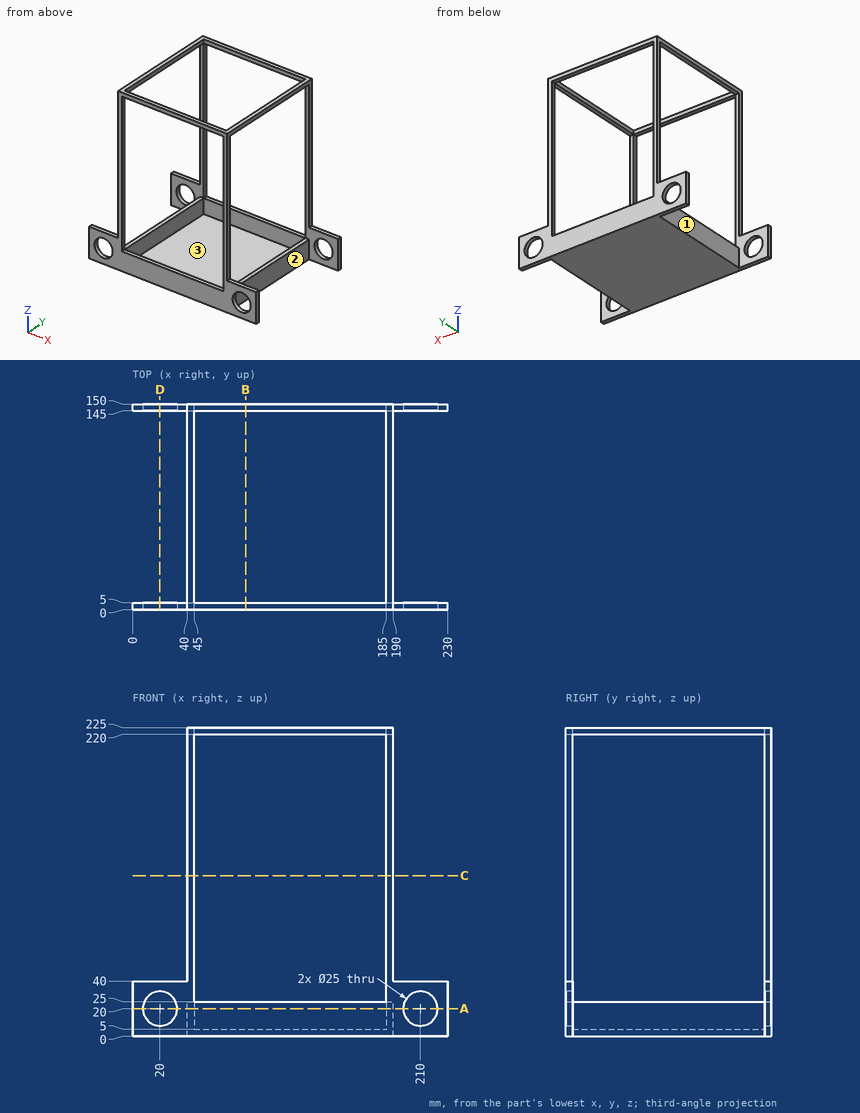
The drawing under review shows one solid part. Ordinate dimensions are in mm from its lowest x, y, z. Coordinates: 2 decimals unless noted, no trailing zeros. Loops run counter-clockwise (first coordinate to the right, second up) from the corner with the lowest first, then second, coordinate; pieces in that order, holes last. Notation, with made-up numbers: M 84.25,27.25 L 109.25,27.25 A22 ccw 109.25,56.25 Z; hole C -15.5,86 d11. An arc over 180 degrees is marked long. Use one line per item in the form item = value.
(1) For line 1 along X through (y, z) = (1, 20); line 2 along X through (y, z) = (55, 18.5); line 3 along Y through (x, z) = (73.5, 15.5), list the stretches that pass through material, from the lowest coordinate up. Write a range as from..to.
Return value:
line_1 = 0..7.5, 32.5..197.5, 222.5..230
line_2 = 40..45, 185..190
line_3 = 0..5, 145..150
(2) Consider section A-A (z = 20). Give the number of separate pieces and of enclosed holes in the cut face, and give its area (3 significant figures).
Return value:
separate_pieces = 5
enclosed_holes = 1
area = 3,200 mm2
(3) Consider section C-C (z = 117). Write out the cut boundary in (x, y), and give its area (3 significant figures).
Return value:
outline = M 40,0 L 45,0 L 45,5 L 40,5 Z; M 40,145 L 45,145 L 45,150 L 40,150 Z; M 185,0 L 190,0 L 190,5 L 185,5 Z; M 185,145 L 190,145 L 190,150 L 185,150 Z
area = 100 mm2
(4) Draft analysis for pull direction X (two halves, no side actions). For the marked faces 1, 2 and 3, state which applies: pulls with the +X half, pulls with the -X half, needs draft (parallel to the pull), parting line crosses it, or undercut.
Return value:
face_1 = pulls with the -X half
face_2 = pulls with the +X half
face_3 = undercut
(5) Clearance check with flat-ended pins moving along their axes: P1, Ø20, axis at y = 76.5, z = 17.5, coming from the +X side; P2, Ø5.5, axis at x = 210, y = 2, coming from the +Z side; P3, Ø4, axis at y = 147.5, z = 101, coming from the -X side. State where each tip first meets the part, or that it passes through.
Return value:
P1 = 190
P2 = 40
P3 = 40
(6) Consider section B-B (x = 82.5). Write out the cut boundary in (y, z), and give its area (3 significant figures).
Return value:
outline = M 0,0 L 150,0 L 150,25 L 145,25 L 145,5 L 5,5 L 5,25 L 0,25 Z; M 0,220 L 5,220 L 5,225 L 0,225 Z; M 145,220 L 150,220 L 150,225 L 145,225 Z
area = 1,000 mm2
(7) Consider section D-D (x = 20). Write out the cut boundary in (y, z), and give its area (3 significant figures).
Return value:
outline = M 0,0 L 5,0 L 5,7.5 L 0,7.5 Z; M 0,32.5 L 5,32.5 L 5,40 L 0,40 Z; M 145,0 L 150,0 L 150,7.5 L 145,7.5 Z; M 145,32.5 L 150,32.5 L 150,40 L 145,40 Z
area = 150 mm2
